Geometry: final body of the model. Coordinates: model frame, mm. A direction names the side the tool comes from. Coordinates: 2 decimals unless noted, no trailing zeros. Write each loop counter-clockwise with the first axis right and the second up, starting at its lowest first coordinate (ties: lowest second). Pieces come first, ordered by that corner, then holes. Notation, with made-up numbers: (25, 27.5) -> (61, 27.5) arc R33 ccw to (61, 56.5) -> close; hole circle Ø4 at (82.5, 1). An arc over 180 degrees is marked (long way). One line per item, written item: value.
```python
from build123d import *

# Parameters (mm, degrees)
SKETCH_1_R       = 2.7
SKETCH_1_R_2     = 2.2
EXTRUDE_1_DEPTH  = 5
SKETCH_1_4_W     = 29.632105645
SKETCH_1_4_H     = 2
EXTRUDE_2_DEPTH  = 6.8
CHAMFER_1_SIZE   = 3
CHAMFER_1_SIZE_2 = 6.8
CHAMFER_2_SIZE   = 3
CHAMFER_2_SIZE_2 = 6.8


with BuildPart() as part:
    # 草图1 → 凸台-拉伸1 (new body)
    with BuildSketch(Plane.XY):
        with BuildLine():
            Line((-22.305856328, 31.375150719), (-46.237237552, 8.916767146))
            ThreePointArc((-46.237237552, 8.916767146), (-47.170759472, 7.589190013), (-47.5, 6))
            Line((-47.5, 6), (-47.5, -6))
            ThreePointArc((-47.5, -6), (-47.170759472, -7.589190013), (-46.237237552, -8.916767146))
            Line((-46.237237552, -8.916767146), (-22.305856328, -31.375150719))
            ThreePointArc((-22.305856328, -31.375150719), (-19.495338483, -32.858506483), (-16.321429443, -32.698330691))
            Line((-16.321429443, -32.698330691), (20.078570557, -20.698330691))
            ThreePointArc((20.078570557, -20.698330691), (23.061657297, -18.516288999), (24.2, -15))
            Line((24.2, -15), (24.2, 15))
            ThreePointArc((24.2, 15), (23.061657297, 18.516288999), (20.078570557, 20.698330691))
            Line((20.078570557, 20.698330691), (-16.321429443, 32.698330691))
            ThreePointArc((-16.321429443, 32.698330691), (-19.495338483, 32.858506483), (-22.305856328, 31.375150719))
        make_face()
        with Locations((18.2, -15)):
            Circle(SKETCH_1_R, mode=Mode.SUBTRACT)
        with Locations((-38, 0)):
            Circle(SKETCH_1_R_2, mode=Mode.SUBTRACT)
        with Locations((-18, 0)):
            Circle(SKETCH_1_R_2, mode=Mode.SUBTRACT)
        with Locations((-18.2, 27)):
            Circle(SKETCH_1_R, mode=Mode.SUBTRACT)
        with Locations((18.2, 15)):
            Circle(SKETCH_1_R, mode=Mode.SUBTRACT)
        with Locations((-18.2, -27)):
            Circle(SKETCH_1_R, mode=Mode.SUBTRACT)
    extrude(amount=EXTRUDE_1_DEPTH)

    # 草图4 → 旋转1 (revolve)
    with BuildSketch(Plane(origin=(6.244417819, 18.941400719, 0), x_dir=(-0.9497217817885489, 0.3130950928973239, 0), z_dir=(-0.3130950928973239, -0.9497217817885489, 0)), mode=Mode.PRIVATE) as revolve_1_sk:
        Polygon((-6.588510035, 0), (-7.588510035, 8.7), (-9.888510035, 8.7), (-9.888510035, 0), align=None)
    revolve_1 = revolve(revolve_1_sk.sketch.rotate(Axis((18.2, 15, 4.45283877), (0, 0, -1)), 161.754145472), axis=Axis((18.2, 15, 4.45283877), (0, 0, -1)))

    # 草图4<3> → 旋转2 (revolve)
    with BuildSketch(Plane(origin=(6.244417819, 18.941400719, 0), x_dir=(-0.9497217817885489, 0.3130950928973239, 0), z_dir=(-0.3130950928973239, -0.9497217817885489, 0)), mode=Mode.PRIVATE) as revolve_2_sk:
        Polygon((30.738503937, 8.7), (28.438503937, 8.7), (28.438503937, 0), (31.738503937, 0), align=None)
    revolve_2 = revolve(revolve_2_sk.sketch.rotate(Axis((-18.2, 27, 0), (0, 0, -1)), 161.754145472), axis=Axis((-18.2, 27, 0), (0, 0, -1)))

    # 镜向1: 旋转1, 旋转2 across plane
    add(revolve_1.mirror(Plane.ZX))
    add(revolve_2.mirror(Plane.ZX))

    # 草图1<4> → 凸台-拉伸2 (add)
    with BuildSketch(Plane.XY):
        with Locations((-27.816052823, 11.3)):
            Rectangle(SKETCH_1_4_W, SKETCH_1_4_H)
        with Locations((-27.816052823, -11.3)):
            Rectangle(SKETCH_1_4_W, SKETCH_1_4_H)
    extrude(amount=-EXTRUDE_2_DEPTH)

    # 倒角1
    # the kernel refuses this chamfer: 6.8, 3 mm, written as the material it adds along each edge
    with BuildSketch(Plane(origin=(-13, 12.3, 0), x_dir=(0, 0.9968133817371192, 0.07976892872421078), z_dir=(-1, 0, 0))) as chamfer_1_piece_1_section:
        Polygon((CHAMFER_1_SIZE * 0.996813381737, CHAMFER_1_SIZE * 0.0797689287242), (-CHAMFER_1_SIZE_2 * 0.0797689287242, CHAMFER_1_SIZE_2 * 0.996813381737), (0, 0), align=None)
    chamfer_1_piece_1 = extrude(amount=29.632105645, mode=Mode.PRIVATE)
    chamfer_1_piece_1 = split(chamfer_1_piece_1, bisect_by=Plane(origin=(-34.029834246, 20.372793997, -2.314232385), z_dir=(0.6843093880009448, -0.7291917864963733, 0)), keep=Keep.TOP, mode=Mode.PRIVATE)
    chamfer_1_piece_1 = split(chamfer_1_piece_1, bisect_by=Plane(origin=(-27.32033499, 13.223232944, -6.8), z_dir=(0, 0, 1)), keep=Keep.TOP, mode=Mode.PRIVATE)
    add(chamfer_1_piece_1)

    # 倒角2
    # the kernel refuses this chamfer: 6.8, 3 mm, written as the material it adds along each edge
    with BuildSketch(Plane(origin=(-42.632105645, -12.3, 0), x_dir=(0, -0.9968133817371192, 0.07976892872421078), z_dir=(1, 0, 0))) as chamfer_2_piece_1_section:
        Polygon((CHAMFER_2_SIZE * 0.996813381737, CHAMFER_2_SIZE * 0.0797689287242), (-CHAMFER_2_SIZE_2 * 0.0797689287242, CHAMFER_2_SIZE_2 * 0.996813381737), (0, 0), align=None)
    chamfer_2_piece_1 = extrude(amount=29.632105645, mode=Mode.PRIVATE)
    chamfer_2_piece_1 = split(chamfer_2_piece_1, bisect_by=Plane(origin=(-34.029834246, -20.372793997, -2.314232385), z_dir=(0.6843093880009445, 0.7291917864963735, 0)), keep=Keep.TOP, mode=Mode.PRIVATE)
    chamfer_2_piece_1 = split(chamfer_2_piece_1, bisect_by=Plane(origin=(-27.32033499, -13.223232944, -6.8), z_dir=(0, 0, 1)), keep=Keep.TOP, mode=Mode.PRIVATE)
    add(chamfer_2_piece_1)


solid = part.part
```
(1) Line query: line 1 (Y direction, x = -18, z = 3.95); line 2 (X direction, y = -1.5, z = 3.25); line 3 (Y direction, x = -18.2, z = -5). Output: solid intervals per line, ascending. Write a range as [from, to].
Responses:
line 1: y = [-33, -29.69], [-24.31, -2.2], [2.2, 24.31], [29.69, 33]
line 2: x = [-47.5, -39.61], [-36.39, -19.61], [-16.39, 24.2]
line 3: y = [-32.43, -29.7], [-24.3, -21.57], [-13.09, -10.3], [10.3, 13.09], [21.57, 24.3], [29.7, 32.43]
(2) Section A-A (y = 0). Return the cut outline in (x, z).
Responses:
outline: (-47.5, 0) -> (-40.2, 0) -> (-40.2, 5) -> (-47.5, 5) -> close; (-35.8, 0) -> (-20.2, 0) -> (-20.2, 5) -> (-35.8, 5) -> close; (-15.8, 0) -> (24.2, 0) -> (24.2, 5) -> (-15.8, 5) -> close
(3) Section B-B (z = -5.25). State how many separate pieces and enclosed holes the cut face has, then the cut area to 3 significant figures.
Responses:
separate pieces: 6
enclosed holes: 4
area: 433 mm2
(4) Pull-direction query (X, two-part tool) for faces 4 (the flat face through (20.4, 17.2, -8.7)), 5 (the flat face through (-13, -12, -3)), 6 (the flat face through (-42.632, 11, -3)); classes: released by +X, released by -X, zero draft, split by the parting line, or undercut.
Responses:
face 4: zero draft
face 5: undercut
face 6: released by -X
(5) First-contact query: pin 1 (7 mm diameter, centred on x = -38, y = 0, fed in from -Z); pin 2 (0.6 mm diameter, centred on y = -11.5, z = -4, fed in from -X); pin 3 (5.5 mm diameter, centred on y = 12.5, z = -3, fed in from +X). Flat tips, straight axial feed; report the tip coordinate or a pass-through.
Responses:
pin 1: stops at z = 0
pin 2: stops at x = -42.63
pin 3: stops at x = 24.05
(6) Section C-C (z = 1.5). Return the cut outline in (x, y).
Responses:
outline: (-47.5, -6) arc R4 ccw to (-46.24, -8.92) -> (-22.31, -31.38) arc R6 ccw to (-16.32, -32.7) -> (20.08, -20.7) arc R6 ccw to (24.2, -15) -> (24.2, 15) arc R6 ccw to (20.08, 20.7) -> (-16.32, 32.7) arc R6 ccw to (-22.31, 31.38) -> (-46.24, 8.92) arc R4 ccw to (-47.5, 6) -> close; hole circle Ø4.4 at (-38, 0); hole circle Ø5.4 at (-18.2, -27); hole circle Ø5.4 at (-18.2, 27); hole circle Ø4.4 at (-18, 0); hole circle Ø5.4 at (18.2, -15); hole circle Ø5.4 at (18.2, 15)
(7) Reachability of faces 1 (the cylindrical face through (-19.45, 32.87, 2.46)), 2 (the flat face through (-28, -13.8, -3.4)), 3 (the flat face through (-4, 0, 0)) from +Z, -Z, +X, -X, +Y, -Y: full face, straight path, thin tool, end or side. Return the list, or none.
Responses:
face 1: +Z, -Z, +Y
face 2: -Z, -X
face 3: -Z
